from build123d import *

# Parameters (mm, degrees)
SKETCH1_R           = 2.8
BOSS_EXTRUDE1_DEPTH = 1.5
SKETCH2_R           = 1.5
BOSS_EXTRUDE2_DEPTH = 35
CHAMFER1_SIZE       = 0.5
CHAMFER2_SIZE       = 0.5


with BuildPart() as part:
    # Sketch1 → Boss-Extrude1 (new body, symmetric)
    with BuildSketch(Plane(origin=(0, 0, 0), x_dir=(1, 0, 0), z_dir=(0, 1, 0))):
        Circle(SKETCH1_R)
    extrude(amount=BOSS_EXTRUDE1_DEPTH, both=True)

    # Sketch2 → Boss-Extrude2 (add)
    with BuildSketch(Plane(origin=(0, 1.5, 0), x_dir=(1, 0, 0), z_dir=(0, 1, 0))):
        Circle(SKETCH2_R)
    extrude(amount=BOSS_EXTRUDE2_DEPTH)

    # Chamfer1
    chamfer1_edges = [part.edges().sort_by_distance(p)[0] for p in [
        (-1.5, 36.5, 0),
    ]]
    chamfer(chamfer1_edges, length=CHAMFER1_SIZE)

    # Chamfer2
    chamfer2_edges = [part.edges().sort_by_distance(p)[0] for p in [
        (-2.8, -1.5, 0),
        (-2.8, 1.5, 0),
    ]]
    chamfer(chamfer2_edges, length=CHAMFER2_SIZE)


solid = part.part
The model under review builds one solid part; all positions refer to its coordinate system, in mm. A direction names the side the tool comes from. Coordinates: 2 decimals unless noted, no trailing zeros. Loops run counter-clockwise (first coordinate to the right, second up) from the corner with the lowest first, then second, coordinate; pieces in that order, holes last. Notation, with made-up numbers: (31.25, 60) -> (40.25, 60) arc R18 cw to (40.25, 87) -> close; hole circle Ø6 at (-17.75, 51.25). An arc over 180 degrees is marked (long way). Use a Markdown table: item, result. Add a question column.
1. Add section A-A on z = 0. Write out the cut boundary in (x, y).
2. Clearance check with flat-ended pins moving along their axes: pin 1 Ø1 at (y, z) = (21, 1) entering from +X; pin 2 Ø2 at (x, z) = (-2, -0.5) entering from +Y; pin 3 Ø1.5 at (x, y) = (-1.5, 18) entering from -Z. State where each tip first meets the part, or that it passes through.
3. Add section B-B on x = 0. Write out the cut boundary in (y, z), plus the area to 3 significant figures.
4. To check wall thickness, follow line 1 (Y direction, x = -0.5, z = -1.8); line 2 (Z direction, x = -0.3, y = 12); line 3 (X direction, y = 35.5, z = 0.65). State the ranges of each line that lie inside material, in increasing order.
5. Machinability: for faces 1 (the face through (0, -1.5, 0)), 2 (the face through (0, 1.5, 2)), which of the approach directions +Z, -Z, +X, -X, +Y, -Y give a long, thin tool a straight path to every point of the face, cutting with its end or side? Answer none if there is none.
6. Add section C-C on y = 27. Write out the cut boundary in (x, z).
Returned:
| question | item | result |
|---|---|---|
| 1 | outline | (-2.8, -1) -> (-2.3, -1.5) -> (2.3, -1.5) -> (2.8, -1) -> (2.8, 1) -> (2.3, 1.5) -> (1.5, 1.5) -> (1.5, 36) -> (1, 36.5) -> (-1, 36.5) -> (-1.5, 36) -> (-1.5, 1.5) -> (-2.3, 1.5) -> (-2.8, 1) -> close |
| 2 | pin 1 | stops at x = 1.41 |
| 2 | pin 2 | stops at y = 36.44 |
| 2 | pin 3 | stops at z = -1.3 |
| 3 | outline | (-1.5, -2.3) -> (-1, -2.8) -> (1, -2.8) -> (1.5, -2.3) -> (1.5, -1.5) -> (36, -1.5) -> (36.5, -1) -> (36.5, 1) -> (36, 1.5) -> (1.5, 1.5) -> (1.5, 2.3) -> (1, 2.8) -> (-1, 2.8) -> (-1.5, 2.3) -> close |
| 3 | area | 121 mm² |
| 4 | line 1 | y = -1.5 to 1.5 |
| 4 | line 2 | z = -1.47 to 1.47 |
| 4 | line 3 | x = -1.35 to 1.35 |
| 5 | face 1 | +Z, -Z, +X, -X, -Y |
| 5 | face 2 | +Y |
| 6 | outline | circle Ø3 at (0, 0) |
